from build123d import *

# Parameters (mm, degrees)
SKETCH_W     = 10
SKETCH_H     = 25
SKETCH_R     = 1.75
PAD_DEPTH    = 1.5
SKETCH001_W  = 5
SKETCH001_H  = 5
PAD001_DEPTH = 0.5
SKETCH002_W  = 4
SKETCH002_H  = 6
PAD002_DEPTH = 7


with BuildPart() as part:
    # Sketch → Pad (new body)
    with BuildSketch(Plane.XZ):
        Rectangle(SKETCH_W, SKETCH_H)
        with Locations((0, -2)):
            Circle(SKETCH_R, mode=Mode.SUBTRACT)
    extrude(amount=PAD_DEPTH)

    # Sketch001 (on Face7 of Pad) → Pad001 (join)
    with BuildSketch(Plane.XZ.offset(1.5)):
        with Locations((0, 8)):
            Rectangle(SKETCH001_W, SKETCH001_H)
    extrude(amount=PAD001_DEPTH)

    # Sketch002 (on Face4 of Pad001) → Pad002 (join)
    with BuildSketch(Plane(origin=(0, 0, 0), x_dir=(1, 0, 0), z_dir=(0, 1, 0))):
        with Locations((0, 9.5)):
            Rectangle(SKETCH002_W, SKETCH002_H)
    extrude(amount=PAD002_DEPTH)


solid = part.part
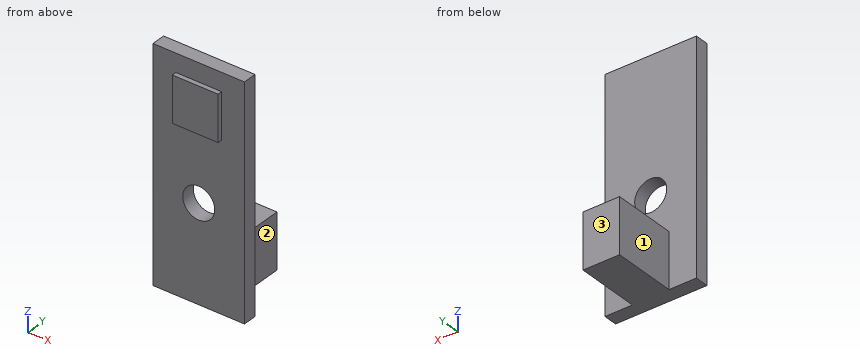
The model under review builds one solid part; all positions refer to its coordinate system, in mm. Face numbers are marked on the shaded views. A direction names the side the tool comes from. Round coordinates to 2 decimals unless told otherwise and drop trailing zeros. Write each loop counter-clockwise with the first axis right and the second up, starting at its lowest first coordinate (ties: lowest second). Pieces come first, ordered by that corner, then holes. Notation, with made-up numbers: M 17.25,5 L 64.25,5 A31 ccw 64.25,43 Z; hole C 77,-18 d7. An arc over 180 degrees is marked long. Use a Markdown table: item, result. Add a question column.
Q1. We need section D-D, the plane y = -1. State the section outline as (x, z) points, plus the area to 3 significant figures.
Q2. Machinability: for the marked faces 1, 2 and 3, which of the approach directions +Z, -Z, +X, -X, +Y, -Y give a long, thin tool a straight path to every point of the face, cutting with its end or side? Answer none if there is none.
Q3. To check wall thickness, follow line 1 (Z direction, x = 0, y = -0.8); line 2 (Y direction, x = 0, z = 2); line 3 (Y direction, x = 0.5, z = 7). State the ranges of each line that lie inside material, in increasing order.
Q4. We need section C-C, the plane z = -6.75. State the section outline as (x, y) points.
Q5. We need section A-A, the plane x = 0. State the section outline as (y, z) points.
Q6. Insertion check: pin 1 (3 mm diameter, centred on x = -2.5, z = -2.5, fed in from -Y); pin 2 (2 mm diameter, centred on x = -0.5, y = 2, fed in from +Z); pin 3 (3 mm diameter, centred on x = 2.5, z = 6, fed in from +Y). Each pin has a flat end and moves straight along its axis. Give the tip position at first contact, or say it passes through.
Q7. We need section B-B, the plane z = -2. State the section outline as (x, y) points, plus the area to 3 significant figures.
Findings below:
| question | item | result |
|---|---|---|
| 1 | outline | M -5,-12.5 L 5,-12.5 L 5,12.5 L -5,12.5 Z; hole C 0,-2 d3.5 |
| 1 | area | 240 mm² |
| 2 | face 1 | +Z, -Z, -X, +Y |
| 2 | face 2 | +Z, -Z, +X, +Y |
| 2 | face 3 | +Z, -Z, +X, -X, +Y |
| 3 | line 1 | z = -12.5 to -3.75, -0.25 to 12.5 |
| 3 | line 2 | y = -1.5 to 0 |
| 3 | line 3 | y = -2 to 0 |
| 4 | outline | M -5,-1.5 L 5,-1.5 L 5,0 L 2,0 L 2,7 L -2,7 L -2,0 L -5,0 Z |
| 5 | outline | M -2,5.5 L -1.5,5.5 L -1.5,-0.25 L 0,-0.25 L 0,12.5 L -1.5,12.5 L -1.5,10.5 L -2,10.5 Z; M -1.5,-12.5 L 7,-12.5 L 7,-6.5 L 0,-6.5 L 0,-3.75 L -1.5,-3.75 Z |
| 6 | pin 1 | stops at y = -1.5 |
| 6 | pin 2 | stops at z = -6.5 |
| 6 | pin 3 | stops at y = 0 |
| 7 | outline | M -5,-1.5 L -1.75,-1.5 L -1.75,0 L -5,0 Z; M 1.75,-1.5 L 5,-1.5 L 5,0 L 1.75,0 Z |
| 7 | area | 9.75 mm² |
